```python
from build123d import *

# Parameters (mm, degrees)
EXTRUDE_1_DEPTH     = 3
SKETCH_2_R          = 1.525
SKETCH_2_R_2        = 1.55
CUT_EXTRUDE_1_DEPTH = 326.276245137
SKETCH_3_R          = 1.55
CUT_EXTRUDE_2_DEPTH = 326.276245137


with BuildPart() as part:
    # 草图1 → 凸台-拉伸1 (new body)
    with BuildSketch(Plane.XY):
        with BuildLine():
            Line((63.562092344, 7.87386317), (63.562092344, 94.767111078))
            Line((63.562092344, 94.767111078), (63.562092344, 159.160358986))
            ThreePointArc((63.562092344, 159.160358986), (64.30521832, 162.943252496), (66.424149005, 166.163912719))
            ThreePointArc((66.424149005, 166.163912719), (68.921247911, 173.655107589), (64.550802827, 180.231787094))
            ThreePointArc((64.550802827, 180.231787094), (63.826785594, 180.962931434), (63.562092344, 181.957270653))
            Line((63.562092344, 181.957270653), (63.562092344, 242.267111078))
            ThreePointArc((63.562092344, 242.267111078), (66.491024532, 249.33817889), (73.562092344, 252.267111078))
            Line((73.562092344, 252.267111078), (118, 252.267111078))
            ThreePointArc((118, 252.267111078), (119.414213562, 252.852897516), (120, 254.267111078))
            Line((120, 254.267111078), (120, 262.267111078))
            ThreePointArc((120, 262.267111078), (119.414213562, 263.681324641), (118, 264.267111078))
            Line((118, 264.267111078), (39.254483947, 264.267111078))
            ThreePointArc((39.254483947, 264.267111078), (32.183416135, 267.196043266), (29.254483947, 274.267111078))
            Line((29.254483947, 274.267111078), (29.254483947, 300.317111078))
            ThreePointArc((29.254483947, 300.317111078), (28.668697509, 301.731324641), (27.254483947, 302.317111078))
            Line((27.254483947, 302.317111078), (19.254483947, 302.317111078))
            Line((19.254483947, 302.317111078), (15.254483947, 302.317111078))
            Line((15.254483947, 302.317111078), (-28.745516053, 302.317111078))
            ThreePointArc((-28.745516053, 302.317111078), (-30.159729616, 301.731324641), (-30.745516053, 300.317111078))
            Line((-30.745516053, 300.317111078), (-30.745516053, 274.267111078))
            ThreePointArc((-30.745516053, 274.267111078), (-33.674448242, 267.196043266), (-40.745516053, 264.267111078))
            Line((-40.745516053, 264.267111078), (-50.745516053, 264.267111078))
            Line((-50.745516053, 264.267111078), (-118, 264.267111078))
            ThreePointArc((-118, 264.267111078), (-119.414213562, 263.681324641), (-120, 262.267111078))
            Line((-120, 262.267111078), (-120, 254.267111078))
            ThreePointArc((-120, 254.267111078), (-119.414213562, 252.852897516), (-118, 252.267111078))
            Line((-118, 252.267111078), (-96, 252.267111078))
            ThreePointArc((-96, 252.267111078), (-88.928932188, 249.33817889), (-86, 242.267111078))
            Line((-86, 242.267111078), (-86, 180.016945513))
            ThreePointArc((-86, 180.016945513), (-86.141359245, 179.278396568), (-86.545454545, 178.644248343))
            ThreePointArc((-86.545454545, 178.644248343), (-88.927223928, 173.609333888), (-87.889845719, 168.136945432))
            ThreePointArc((-87.889845719, 168.136945432), (-86.47997992, 164.570466876), (-86, 160.765587097))
            Line((-86, 160.765587097), (-86, 6.26863506))
            ThreePointArc((-86, 6.26863506), (-86.47997992, 2.46375528), (-87.889845719, -1.102723275))
            ThreePointArc((-87.889845719, -1.102723275), (-85.757688337, -12.35018789), (-74.310049328, -12.406013139))
            ThreePointArc((-74.310049328, -12.406013139), (-73.716746861, -12.071562552), (-73.045615845, -11.955596298))
            Line((-73.045615845, -11.955596298), (52.949414819, -11.955596298))
            ThreePointArc((52.949414819, -11.955596298), (53.472168985, -12.02512276), (53.958577903, -12.228868216))
            ThreePointArc((53.958577903, -12.228868216), (54.359402341, -12.475964985), (54.748150651, -12.741656151))
            ThreePointArc((54.748150651, -12.741656151), (66.831176576, -11.292498685), (66.424149005, 0.870309438))
            ThreePointArc((66.424149005, 0.870309438), (64.30521832, 4.090969661), (63.562092344, 7.87386317))
        make_face()
        with BuildLine():
            Line((-74, 150.511247137), (-74, 10.044403702))
            ThreePointArc((-74, 10.044403702), (-71.071067812, 2.97333589), (-64, 0.044403702))
            Line((-64, 0.044403702), (40.00099757, 0.044403702))
            ThreePointArc((40.00099757, 0.044403702), (41.791102309, 1.152481605), (41.597631541, 3.248878676))
            Line((41.597631541, 3.248878676), (-70.403366029, 151.715722111))
            ThreePointArc((-70.403366029, 151.715722111), (-72.635111037, 152.407726499), (-74, 150.511247137))
        make_face(mode=Mode.SUBTRACT)
        with BuildLine():
            Line((51.562092344, 137.909223904), (51.562092344, 110.767111078))
            ThreePointArc((51.562092344, 110.767111078), (48.633160156, 103.696043266), (41.562092344, 100.767111078))
            Line((41.562092344, 100.767111078), (-14.286066222, 100.767111078))
            Line((-14.286066222, 100.767111078), (-59.531026404, 164.754540121))
            ThreePointArc((-59.531026404, 164.754540121), (-59.674164346, 166.828634703), (-57.898021395, 167.909223904))
            Line((-57.898021395, 167.909223904), (21.562092344, 167.909223904))
            ThreePointArc((21.562092344, 167.909223904), (42.77529578, 159.12242734), (51.562092344, 137.909223904))
        make_face(mode=Mode.SUBTRACT)
        with BuildLine():
            Line((47.929087335, 12.779682035), (-5.800969535, 88.767111078))
            Line((-5.800969535, 88.767111078), (41.562092344, 88.767111078))
            ThreePointArc((41.562092344, 88.767111078), (48.633160156, 85.83817889), (51.562092344, 78.767111078))
            Line((51.562092344, 78.767111078), (51.562092344, 13.934365818))
            ThreePointArc((51.562092344, 13.934365818), (50.167893459, 12.028321483), (47.929087335, 12.779682035))
        make_face(mode=Mode.SUBTRACT)
        with BuildLine():
            Line((17.562092344, 242.267111078), (17.562092344, 189.673981411))
            ThreePointArc((17.562092344, 189.673981411), (20.491024532, 182.602913599), (27.562092344, 179.673981411))
            Line((27.562092344, 179.673981411), (41.562092344, 179.673981411))
            ThreePointArc((41.562092344, 179.673981411), (48.633160156, 182.602913599), (51.562092344, 189.673981411))
            Line((51.562092344, 189.673981411), (51.562092344, 242.267111078))
            ThreePointArc((51.562092344, 242.267111078), (48.633160156, 249.33817889), (41.562092344, 252.267111078))
            Line((41.562092344, 252.267111078), (27.562092344, 252.267111078))
            ThreePointArc((27.562092344, 252.267111078), (20.491024532, 249.33817889), (17.562092344, 242.267111078))
        make_face(mode=Mode.SUBTRACT)
        with BuildLine():
            Line((-40, 242.267111078), (-40, 188.467111078))
            ThreePointArc((-40, 188.467111078), (-42.928932188, 181.396043266), (-50, 178.467111078))
            Line((-50, 178.467111078), (-64, 178.467111078))
            ThreePointArc((-64, 178.467111078), (-71.071067812, 181.396043266), (-74, 188.467111078))
            Line((-74, 188.467111078), (-74, 242.267111078))
            ThreePointArc((-74, 242.267111078), (-71.071067812, 249.33817889), (-64, 252.267111078))
            Line((-64, 252.267111078), (-50, 252.267111078))
            ThreePointArc((-50, 252.267111078), (-42.928932188, 249.33817889), (-40, 242.267111078))
        make_face(mode=Mode.SUBTRACT)
    extrude(amount=-EXTRUDE_1_DEPTH)

    # 草图2 → 切除-拉伸1 (cut, through all)
    with BuildSketch(Plane(origin=(0, 0, -3), x_dir=(-1, 0, 0), z_dir=(0, 0, -1))):
        with Locations((-60, 172.467111078)):
            Circle(SKETCH_2_R)
        with Locations((-60, -5.432888922)):
            Circle(SKETCH_2_R)
        with Locations((80, -5.432888922)):
            Circle(SKETCH_2_R)
        with Locations((80, 172.467111078)):
            Circle(SKETCH_2_R)
        with Locations((0, 258.267111078)):
            Circle(SKETCH_2_R_2)
        with Locations((-97.15, 258.267111078)):
            Circle(SKETCH_2_R)
        with Locations((97.15, 258.267111078)):
            Circle(SKETCH_2_R)
        with BuildLine():
            Line((28, 233.267111078), (28, 203.267111078))
            ThreePointArc((28, 203.267111078), (11.218953828, 186.486064906), (-5.562092344, 203.267111078))
            Line((-5.562092344, 203.267111078), (-5.562092344, 233.267111078))
            ThreePointArc((-5.562092344, 233.267111078), (11.218953828, 250.04815725), (28, 233.267111078))
        make_face()
    extrude(amount=-CUT_EXTRUDE_1_DEPTH, mode=Mode.SUBTRACT)

    # 草图3 → 切除-拉伸2 (cut, through all)
    with BuildSketch(Plane(origin=(0, 0, -3), x_dir=(-1, 0, 0), z_dir=(0, 0, -1))):
        with Locations((-23.254483947, 296.317111078)):
            Circle(SKETCH_3_R)
        with Locations((24.745516053, 296.317111078)):
            Circle(SKETCH_3_R)
        with Locations((-23.254483947, 289.317111078)):
            Circle(SKETCH_3_R)
        with Locations((24.745516053, 289.317111078)):
            Circle(SKETCH_3_R)
        with Locations((-23.254483947, 282.317111078)):
            Circle(SKETCH_3_R)
        with Locations((24.745516053, 282.317111078)):
            Circle(SKETCH_3_R)
        with BuildLine():
            Line((-4.254483947, 297.817111078), (5.745516053, 297.817111078))
            ThreePointArc((5.745516053, 297.817111078), (7.245516053, 296.317111078), (5.745516053, 294.817111078))
            Line((5.745516053, 294.817111078), (-4.254483947, 294.817111078))
            ThreePointArc((-4.254483947, 294.817111078), (-5.754483947, 296.317111078), (-4.254483947, 297.817111078))
        make_face()
        with BuildLine():
            Line((-4.254483947, 290.817111078), (5.745516053, 290.817111078))
            ThreePointArc((5.745516053, 290.817111078), (7.245516053, 289.317111078), (5.745516053, 287.817111078))
            Line((5.745516053, 287.817111078), (-4.254483947, 287.817111078))
            ThreePointArc((-4.254483947, 287.817111078), (-5.754483947, 289.317111078), (-4.254483947, 290.817111078))
        make_face()
        with BuildLine():
            Line((-4.254483947, 283.817111078), (5.745516053, 283.817111078))
            ThreePointArc((5.745516053, 283.817111078), (7.245516053, 282.317111078), (5.745516053, 280.817111078))
            Line((5.745516053, 280.817111078), (-4.254483947, 280.817111078))
            ThreePointArc((-4.254483947, 280.817111078), (-5.754483947, 282.317111078), (-4.254483947, 283.817111078))
        make_face()
    extrude(amount=-CUT_EXTRUDE_2_DEPTH, mode=Mode.SUBTRACT)


solid = part.part
```
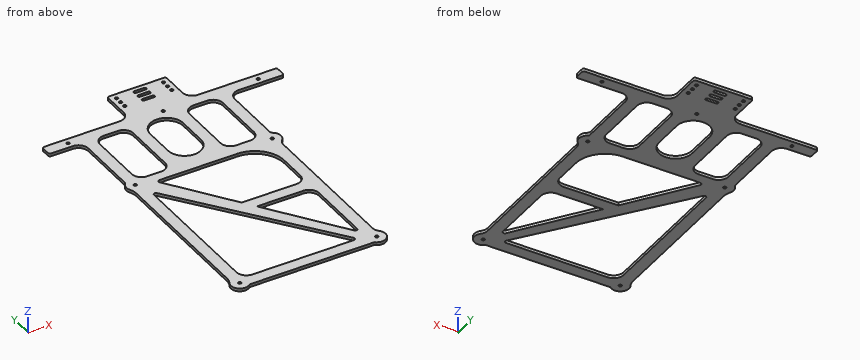
Verification items for the finished model (mm, model axes). Coordinates: 2 decimals unless noted, no trailing zeros. Loops run counter-clockwise (first coordinate to the right, second up) from the corner with the lowest first, then second, coordinate; pieces in that order, holes last. Notation, with made-up numbers: (27.5, 56.5) -> (82.5, 56.5) arc R23 ccw to (82.5, 90.5) -> close; hole circle Ø11 at (35, 52.5). An arc over 180 degrees is marked (long way). Answer in a Markdown table with one row per item.
1) Section check D-D (x = 91.5). Record the cut outline in (y, z), and give its area (3 significant figures).
The answers:
| item | result |
|---|---|
| outline | (252.27, -3) -> (264.27, -3) -> (264.27, 0) -> (252.27, 0) -> close |
| area | 36.0 mm2 |
2) Section check C-C (x = 13). Record the cut outline in (y, z), and give its area (3 significant figures).
The answers:
| item | result |
|---|---|
| outline | (-11.96, -3) -> (0.04, -3) -> (0.04, 0) -> (-11.96, 0) -> close; (41.16, -3) -> (62.18, -3) -> (62.18, 0) -> (41.16, 0) -> close; (88.77, -3) -> (100.77, -3) -> (100.77, 0) -> (88.77, 0) -> close; (167.91, -3) -> (302.32, -3) -> (302.32, 0) -> (167.91, 0) -> close |
| area | 538 mm2 |
3) Section check B-B (y = 29.5). Record the cut outline in (x, z), and give its area (3 significant figures).
The answers:
| item | result |
|---|---|
| outline | (-86, -3) -> (-74, -3) -> (-74, 0) -> (-86, 0) -> close; (21.79, -3) -> (36.11, -3) -> (36.11, 0) -> (21.79, 0) -> close; (51.56, -3) -> (63.56, -3) -> (63.56, 0) -> (51.56, 0) -> close |
| area | 115 mm2 |
4) Scan lines: line 1 along X through (y, z) = (282, -0.85); line 2 along X through (y, z) = (231, -2.85); line 3 along X through (y, z) = (136.5, -2.15). Record each from-to range of solid material in increasing order. Write a range as from..to.
The answers:
| item | result |
|---|---|
| line 1 | x = -30.75..-26.26, -23.23..-7.21, 5.72..21.74, 24.77..29.25 |
| line 2 | x = -86..-74, -40..-28, 5.56..17.56, 51.56..63.56 |
| line 3 | x = -86..-74, -58.92..-39.55, 51.56..63.56 |
5) Section check A-A (y = 228). Record the cut outline in (x, z), and give its area (3 significant figures).
The answers:
| item | result |
|---|---|
| outline | (-86, -3) -> (-74, -3) -> (-74, 0) -> (-86, 0) -> close; (-40, -3) -> (-28, -3) -> (-28, 0) -> (-40, 0) -> close; (5.56, -3) -> (17.56, -3) -> (17.56, 0) -> (5.56, 0) -> close; (51.56, -3) -> (63.56, -3) -> (63.56, 0) -> (51.56, 0) -> close |
| area | 144 mm2 |
6) Depth check by flat-ended pin: P1, Ø1.5, axis at y = 216, z = -2, coming from the -X side; P2, Ø0.9, axis at y = 287, z = -1, coming from the +X side; P3, Ø1, axis at y = 33, z = -1, coming from the +X side. Enter the tip coordinate at first touch or a pass-through.
The answers:
| item | result |
|---|---|
| P1 | stops at x = -86 |
| P2 | stops at x = 29.25 |
| P3 | stops at x = 63.56 |
